Can you work these out from the drawing? Everything is in mm from the part's minimum corner. A direction names the side the tool comes from. Coordinates: 2 decimals unless noted, no trailing zeros. Loops run counter-clockwise (first coordinate to the right, second up) from the corner with the lowest first, then second, coordinate; pieces in that order, holes last. Notation, with made-up numbers: M 49,76 L 85,76 A13 ccw 85,84 Z; hole C 9.5,41.25 d2. An arc over 180 degrees is marked long. Write each question's results on one line, items separated by ' | '.
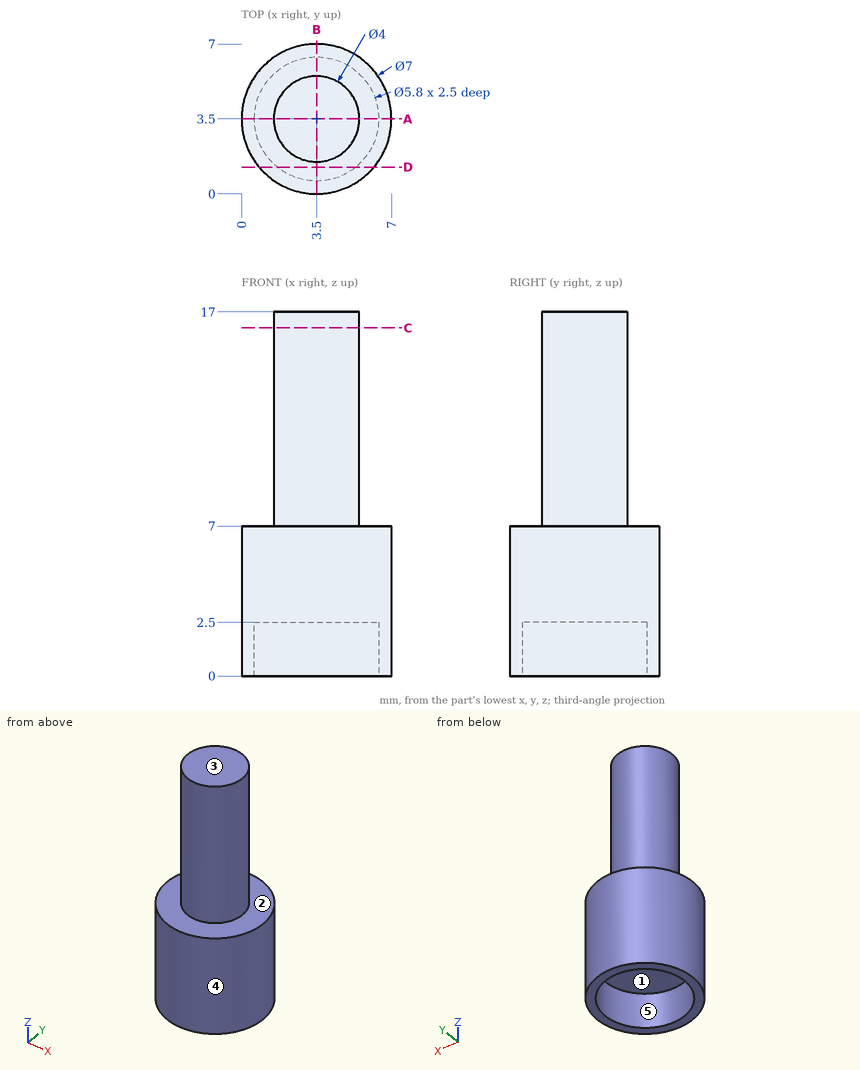
(1) Please list where these lines run through material, in increasing order: probe 1 along Y at (x, z) = (3.5, 0.6); probe 2 along Z at (x, y) = (1.75, 2.75); probe 3 along Z at (x, y) = (2.75, 6.75). Write a range as from..to.
Reported:
probe 1: y = 0..0.6, 6.4..7 | probe 2: z = 2.5..17 | probe 3: z = 0..7
(2) Will these pins go through, and if not, where does the flat tip stop? P1, Ø2, axis at x = 1, z = 2.5, coming from the +Y side; P2, Ø1, axis at y = 2.5, z = 8.5, coming from the -X side; P3, Ø1.7, axis at x = 3.5, y = 4.5, coming from the -Z side.
Reported:
P1: stops at y = 6.66 | P2: stops at x = 1.56 | P3: stops at z = 2.5
(3) Imagine slicing it at D-D, the plane y = 1.25. List the corners of the cut face in (x, z) for me.
Reported:
outline: M 0.82,0 L 1.67,0 L 1.67,2.5 L 5.33,2.5 L 5.33,0 L 6.18,0 L 6.18,7 L 0.82,7 Z
(4) Which directions (+Z, -Z, +X, -X, +Y, -Y) give clear straight access to the entire face, cutting with the end or side of a thin tool? Please do the marked faces 1 and 2.
Reported:
face 1: -Z | face 2: +Z
(5) Imagine slicing it at A-A, the plane y = 3.5. List the corners of the cut face in (x, z) for me.
Reported:
outline: M 0,0 L 0.6,0 L 0.6,2.5 L 6.4,2.5 L 6.4,0 L 7,0 L 7,7 L 5.5,7 L 5.5,17 L 1.5,17 L 1.5,7 L 0,7 Z
(6) If we mould it in two halves opening along X, with no side actions, what happens to the marked faces 3, 4 and 5? For each: released by +X, released by -X, zero draft, split by the parting line, or undercut.
Reported:
face 3: zero draft | face 4: split by the parting line | face 5: undercut
(7) Imagine slicing it at C-C, the plane z = 16.25. List the corners of the cut face in (x, y) for me, and give its area (3 significant figures).
Reported:
outline: C 3.5,3.5 d4 | area: 12.6 mm2
